CAD build for the part. Positions are in the model's coordinates, mm. A direction names the side the tool comes from. Round coordinates to 2 decimals unless told otherwise and drop trailing zeros. Loops run counter-clockwise (first coordinate to the right, second up) from the corner with the lowest first, then second, coordinate; pieces in that order, holes last.
from build123d import *

# Parameters (mm, degrees)
SKETCH1_W               = 39.6
SKETCH1_H               = 14.5
BOSS_EXTRUDE1_DEPTH     = 25
SKETCH2_W               = 40
SKETCH2_H               = 15
BOSS_EXTRUDE2_DEPTH     = 17.3
CUT_EXTRUDE2_DEPTH      = 38.749172176
CUT_EXTRUDE2_DEPTH_BACK = 38.749172176
CHAMFER1_SIZE           = 0.5
CHAMFER2_SIZE           = 0.5
CHAMFER3_SIZE           = 0.5
CHAMFER4_SIZE           = 0.5
LPATTERN2_COUNT         = 2
LPATTERN2_PITCH         = 25
LPATTERN2_COUNT_DIR2    = 2
LPATTERN2_PITCH_DIR2    = 30


with BuildPart() as part:
    # Sketch1 → Boss-Extrude1 (new, symmetric)
    with BuildSketch(Plane(origin=(0, 0, 0), x_dir=(0, 0, -1), z_dir=(1, 0, 0))):
        with Locations((0, 12.25)):
            Rectangle(SKETCH1_W, SKETCH1_H)
    extrude(amount=BOSS_EXTRUDE1_DEPTH, both=True)

    # Sketch2 → Boss-Extrude2 (add, symmetric)
    with BuildSketch(Plane(origin=(0, 0, 0), x_dir=(0, 0, -1), z_dir=(1, 0, 0))):
        with Locations((0, 12.5)):
            Rectangle(SKETCH2_W, SKETCH2_H)
    extrude(amount=BOSS_EXTRUDE2_DEPTH, both=True)

    # Sketch4 → Cut-Extrude2 (cut, two sides: drawn at the far end of the back side and taken through both)
    with BuildSketch(Plane(origin=(0, 0, 0), x_dir=(0, 0, -1), z_dir=(1, 0, 0)).offset(-CUT_EXTRUDE2_DEPTH_BACK)):
        with BuildLine():
            Line((-9.7, 11), (9.7, 11))
            Line((9.7, 11), (10, 10.7))
            Line((10, 10.7), (10, 10.451039482))
            Line((10, 10.451039482), (9.455259378, 10.141421591))
            ThreePointArc((9.455259378, 10.141421591), (8.943868436, 9.701092928), (8.637115571, 9.1))
            Line((8.637115571, 9.1), (7.5, 9.1))
            Line((7.5, 9.1), (7.5, 7.9))
            Line((7.5, 7.9), (8.64, 7.9))
            ThreePointArc((8.64, 7.9), (8.939788863, 7.314120259), (9.434780564, 6.880401858))
            Line((9.434780564, 6.880401858), (10, 6.548960518))
            Line((10, 6.548960518), (10, 0))
            Line((10, 0), (-10, 0))
            Line((-10, 0), (-10, 6.548960518))
            Line((-10, 6.548960518), (-9.434780564, 6.880401858))
            ThreePointArc((-9.434780564, 6.880401858), (-8.939788863, 7.314120259), (-8.64, 7.9))
            Line((-8.64, 7.9), (-7.5, 7.9))
            Line((-7.5, 7.9), (-7.5, 9.1))
            Line((-7.5, 9.1), (-8.637115571, 9.1))
            ThreePointArc((-8.637115571, 9.1), (-8.943868436, 9.701092928), (-9.455259378, 10.141421591))
            Line((-9.455259378, 10.141421591), (-10, 10.451039482))
            Line((-10, 10.451039482), (-10, 10.7))
            Line((-10, 10.7), (-9.7, 11))
        make_face()
    extrude(amount=CUT_EXTRUDE2_DEPTH + CUT_EXTRUDE2_DEPTH_BACK, mode=Mode.SUBTRACT)

    # Chamfer1
    chamfer1_edges = [part.edges().sort_by_distance(p)[0] for p in [
        (-21.15, 19.5, 19.8),
        (-21.15, 19.5, -19.8),
        (21.15, 19.5, 19.8),
        (21.15, 19.5, -19.8),
    ]]
    chamfer(chamfer1_edges, length=CHAMFER1_SIZE)

    # Chamfer2
    chamfer2_edges = [part.edges().sort_by_distance(p)[0] for p in [
        (0, 20, 20),
        (0, 20, -20),
    ]]
    chamfer(chamfer2_edges, length=CHAMFER2_SIZE)

    # Chamfer3
    chamfer3_edges = [part.edges().sort_by_distance(p)[0] for p in [
        (-21.15, 5, -19.8),
        (-21.15, 5, 19.8),
        (21.15, 5, -19.8),
        (21.15, 5, 19.8),
    ]]
    chamfer(chamfer3_edges, length=CHAMFER3_SIZE)

    # Chamfer4
    chamfer4_edges = [part.edges().sort_by_distance(p)[0] for p in [
        (0, 5, 20),
        (0, 5, -20),
    ]]
    chamfer(chamfer4_edges, length=CHAMFER4_SIZE)

    # Sketch7 → Tap2 (revolve, cut)
    with BuildSketch(Plane(origin=(-12.5, 20, -15), x_dir=(0, 0, 1), z_dir=(1, 0, 0))):
        Polygon((0, 0), (0, 8.373995063), (1.621, 7.4), (1.621, 0), align=None)
    tap2 = revolve(axis=Axis((-12.5, 20, -15), (0, -1, 0)), mode=Mode.SUBTRACT)

    # LPattern2: Tap2 2 × 2
    with Locations(*[(i * LPATTERN2_PITCH, 0, j * LPATTERN2_PITCH_DIR2) for i in range(LPATTERN2_COUNT) for j in range(LPATTERN2_COUNT_DIR2) if (i, j) != (0, 0)]):
        add(tap2, mode=Mode.SUBTRACT)


solid = part.part
Item 1: Flat gauge pins, fed straight in: P1, Ø1.9, axis at x = -12.5, z = 15, coming from the +Y side; P2, Ø0.6, axis at x = -7, z = 8, coming from the -Y side. Where does each tip first touch, or does it go through?
Verdict:
P1: stops at y = 12.2
P2: stops at y = 7.9
Item 2: Mould opens along X. For faces 6 (the conical face through (12.221, 11.795, 14.963)), 7 (the flat face through (0, 6, 10)), 8 (the flat face through (-25, 14, 0)) say: released by +X, released by -X, zero draft, split by the parting line, or undercut.
Verdict:
face 6: undercut
face 7: zero draft
face 8: released by -X
Item 3: Cut at A-A (y = 18). List the corners of the cut face in (x, z), plus the area to 3 significant figures.
Verdict:
outline: (-25, -19.8) - (-17.3, -19.8) - (-17.3, -20) - (17.3, -20) - (17.3, -19.8) - (25, -19.8) - (25, 19.8) - (17.3, 19.8) - (17.3, 20) - (-17.3, 20) - (-17.3, 19.8) - (-25, 19.8) - close; hole circle Ø3.24 at (-12.5, -15); hole circle Ø3.24 at (-12.5, 15); hole circle Ø3.24 at (12.5, -15); hole circle Ø3.24 at (12.5, 15)
area: 1,960 mm2
Item 4: 3-axis set-ups, long thin cutter, end or side, ignore diameter. For faces 1 (the flat face through (21, 12, -19.8)), 2 (the flat face through (-21, 19.5, 0)), 3 (the flat face through (0, 9.1, 8)), 4 (the flat face through (21, 19.5, 0)), 5 (the flat face through (-0.4, 8.5, -7.5)): which of +Z, -Z, +X, -X, +Y, -Y reach the whole face in a straight line?
Verdict:
face 1: -Z, +X, +Y, -Y
face 2: +Z, -Z, -X, +Y
face 3: +X, -X
face 4: +Z, -Z, +X, +Y
face 5: +X, -X, -Y
Item 5: Wall check: L1, parallel to X at y = 15, z = -15; L2, parallel to Z at x = 12.5, y = 16.25; L3, parallel to Y at x = -23, z = 14. Give the ranges that are in metal, low to high.
Verdict:
L1: x = -25 to -14.12, -10.88 to 10.88, 14.12 to 25
L2: z = -20 to -16.62, -13.38 to 13.38, 16.62 to 20
L3: y = 5 to 19.5
